The figure shows three views and two pictorial views of one solid part (mm, origin at its lowest corner). Answer the questions. A direction names the side the tool comes from. Coordinates: 2 decimals unless noted, no trailing zeros. Order: outer loops, then holes, each group sorted by start corner. A loop starts at its lowest first (then second) coordinate and runs counter-clockwise, first axis right, second up.
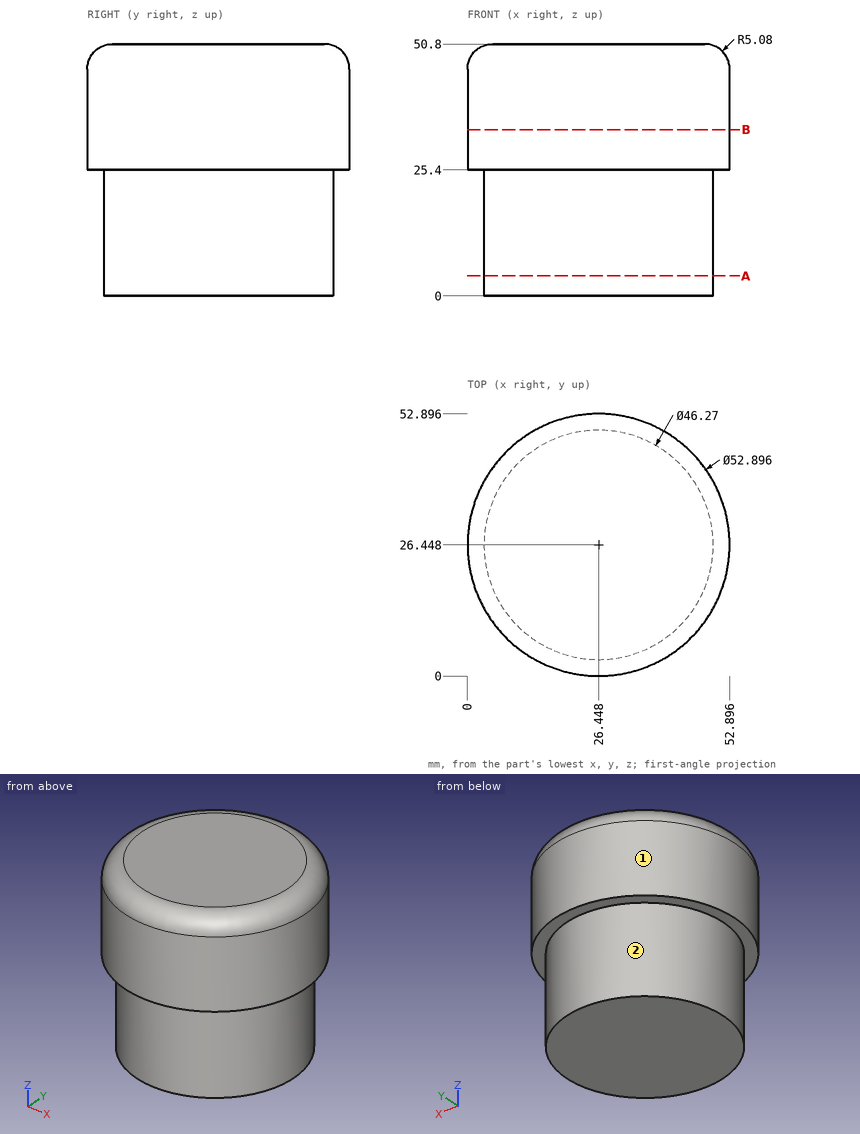
1) A cutting plane is placed at B-B, the plane z = 33.5. Write down the section's boundary in (x, y) (1 decimal).
2) A cutting plane is placed at A-A, the plane z = 4. Write down the section's boundary in (x, y) (1 decimal), plus the area to 3 significant figures.
3) Each of these flat-tipped pins is pushed along its axis until it touches: P1, Ø1, axis at x = 5.5, z = 39.5, coming from the -Y side (1 decimal); P2, Ø6, axis at x = 34, z = 40.5, coming from the -Y side (1 decimal); P3, Ø5, axis at x = 34.5, z = 22.5, coming from the -Y side. Where does it stop, or does it pass through?
4) Straight lines are drawn through the part: probe 1 along X at (y, z) = (27, 40) (1 decimal); probe 2 along X at (y, z) = (41, 45.5) (1 decimal); probe 3 along Y at (x, z) = (7.5, 31) (1 decimal). For each, find the intervals that lie inside material, in ascending order.
5) For the marked faces 1 and 2, determine the directions among +Z, -Z, +X, -X, +Y, -Y from which every point of the face is accessible in a straight line to the end or side of a thin tool.
Working result:
1. outline: circle Ø52.9 at (26.4, 26.4)
2. outline: circle Ø46.3 at (26.4, 26.4)
2. area: 1,680 mm2
3. P1: stops at y = 9.7
3. P2: stops at y = 0.4
3. P3: stops at y = 3.99
4. probe 1: x = 0 to 52.9
4. probe 2: x = 4.4 to 48.5
4. probe 3: y = 8 to 44.9
5. face 1: +Z, -Z
5. face 2: -Z
